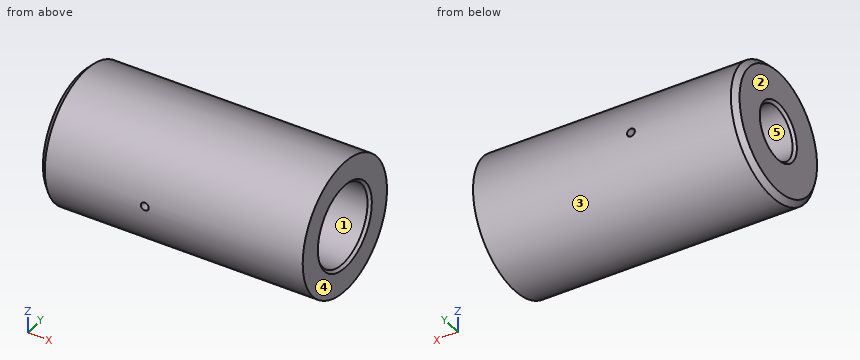
```python
from build123d import *

# Parameters (mm, degrees)
RACCORDO1_R    = 3
SMUSSO1_SIZE   = 2
SMUSSO2_SIZE   = 1
FORO_3_0_3_1_D = 3


with BuildPart() as part:
    # Schizzo2 → Rivoluzione1 (revolve)
    with BuildSketch(Plane.XY, mode=Mode.PRIVATE) as rivoluzione1_sk:
        Polygon((0, 10), (0, 25), (100, 25), (100, 15), (65, 15), (65, 18), (60, 18), (60, 15), (25, 15), (25, 10), align=None)
    revolve(rivoluzione1_sk.sketch.rotate(Axis((0, 0, 0), (1, 0, 0)), 90), axis=Axis((0, 0, 0), (1, 0, 0)))

    # Raccordo1
    raccordo1_edges = [part.edges().sort_by_distance(p)[0] for p in [
        (25, 0, -15),
    ]]
    fillet(raccordo1_edges, radius=RACCORDO1_R)

    # Smusso1
    smusso1_edges = [part.edges().sort_by_distance(p)[0] for p in [
        (0, 0, -25),
    ]]
    chamfer(smusso1_edges, length=SMUSSO1_SIZE)

    # Smusso2
    smusso2_edges = [part.edges().sort_by_distance(p)[0] for p in [
        (100, 0, -15),
        (0, 0, -10),
    ]]
    chamfer(smusso2_edges, length=SMUSSO2_SIZE)

    # Foro Ø3.0 (3)-1 (through all)
    with Locations(Plane(origin=(0, 25, 0), x_dir=(1, 0, 0), z_dir=(0, 1, 0))):
        with Locations((40, 0)):
            Hole(FORO_3_0_3_1_D / 2)


solid = part.part
```
Geometry check sheet. Reference: the model listing, model coordinates, mm. Face numbers are marked on the shaded views. A direction names the side the tool comes from. Give positions to 0.01 mm unless a question says otherwise; leave off trailing zeros. Order: outer loops, then holes, each group sorted by start corner. A loop starts at its lowest first (then second) coordinate and runs counter-clockwise, first axis right, second up. Notation, with made-up numbers: (18.25, 50) - (73.25, 50) arc R27 cw to (73.25, 78) - close; hole circle Ø11 at (-39.75, -32.75). An arc over 180 degrees is marked (long way). Answer in a Markdown table with one row per item. Add a question column.
Q1. Cross-section at B-B, the plane z = 0. Count the separate pieces of the cut face and the enclosed holes in it, then the cut area to 3 significant figures.
Q2. Tool access check on the marked faces 1 and 2. Record the directions out of +Z, -Z, +X, -X, +Y, -Y that give a thin tool (end or side, any length) a straight path to the whole face; none if there is none.
Q3. Cross-section at D-D, the plane x = 6. Enter the section's corners in (y, z).
Q4. Cross-section at A-A, the plane y = 0. Enter the section's corners in (x, z).
Q5. Mould release check, pull along Y, two halves, no side actions. Record for the marked faces 3, 4 and 5: pulls with the +Y half, pulls with the -Y half, needs draft (parallel to the pull), parting line crosses it, or undercut.
Q6. Material ranges on probe 1 along X at (y, z) = (17, -3); probe 2 along Y at (x, z) = (51, 0); probe 3 along Y at (x, z) = (63.65, 0), recorded low to high. Write a range as from..to.
Q7. Gauge pin test, flat ends, axial feed: pin 1 (11 mm diameter, centred on y = -3.5, z = -7.5, fed in from +X); pin 2 (12 mm diameter, centred on x = 29, y = -6.5, fed in from +Z) (3 decimals); pin 3 (24 mm diameter, centred on y = 0, z = 0, fed in from +X); pin 4 (2.5 mm diameter, centred on x = 40, z = 0, fed in from -Y). Record the tip position at first contact, or that the pin passes through.
Q8. Cross-section at C-C, the plane x = 40. Enter the section's corners in (y, z), then the cut area to 3 significant figures.
Check values:
| question | item | result |
|---|---|---|
| 1 | separate pieces | 4 |
| 1 | enclosed holes | 0 |
| 1 | area | 2,160 mm^2 |
| 2 | face 1 | +X |
| 2 | face 2 | +Z, -Z, -X, +Y, -Y |
| 3 | outline | circle Ø50 at (0, 0); hole circle Ø20 at (0, 0) |
| 4 | outline | (0, -23) - (2, -25) - (100, -25) - (100, -16) - (99, -15) - (65, -15) - (65, -18) - (60, -18) - (60, -15) - (28, -15) arc R3 cw to (25, -12) - (25, -10) - (1, -10) - (0, -11) - close; (0, 11) - (1, 10) - (25, 10) - (25, 12) arc R3 cw to (28, 15) - (60, 15) - (60, 18) - (65, 18) - (65, 15) - (99, 15) - (100, 16) - (100, 25) - (2, 25) - (0, 23) - close |
| 5 | face 3 | parting line crosses it |
| 5 | face 4 | needs draft |
| 5 | face 5 | undercut |
| 6 | probe 1 | x = 0..60, 65..100 |
| 6 | probe 2 | y = -25..-15, 15..25 |
| 6 | probe 3 | y = -25..-18, 18..25 |
| 7 | pin 1 | stops at x = 25.58 |
| 7 | pin 2 | stops at z = 24.995 |
| 7 | pin 3 | stops at x = 25 |
| 7 | pin 4 | passes through |
| 8 | outline | (-24.95, -1.5) arc R25 ccw to (24.95, -1.5) - (14.92, -1.5) arc R15 cw to (-14.92, -1.5) - close; (-24.95, 1.5) - (-14.92, 1.5) arc R15 cw to (14.92, 1.5) - (24.95, 1.5) arc R25 ccw to start |
| 8 | area | 1,200 mm^2 |
